Here's how the part is built. I have some questions about the finished solid (model axes, mm). Round coordinates to 2 decimals unless told otherwise and drop trailing zeros. Order: outer loops, then holes, each group sorted by start corner. A loop starts at its lowest first (then second) coordinate and runs counter-clockwise, first axis right, second up. Notation, with made-up numbers: (73, 40.5) - (103, 40.5) arc R30 ccw to (103, 74.5) - close; hole circle Ø1 at (-28, 14.25). An arc over 180 degrees is marked (long way). One line per item, written item: value.
from build123d import *

# Parameters (mm, degrees)
CYLINDER_R     = 5
CYLINDER_DEPTH = 500
BOX_W          = 45
BOX_H          = 45
BOX_DEPTH      = 350


with BuildPart() as screwhole:
    # Cylinder → Cylinder (new body)
    with BuildSketch(Plane(origin=(22.5, 22.5, -150), x_dir=(1, 0, 0), z_dir=(0, 0, 1))):
        Circle(CYLINDER_R)
    extrude(amount=CYLINDER_DEPTH)


with BuildPart() as screwedleg:
    # Box → Box (new body)
    with BuildSketch(Plane.XY):
        with Locations((22.5, 22.5)):
            Rectangle(BOX_W, BOX_H)
    extrude(amount=BOX_DEPTH)

    # Cut: cut ScrewHole
    add(screwhole.part, mode=Mode.SUBTRACT)


solid = screwedleg.part
Q1. If I drill on line 1 along Y through (x, z) = (22.5, 275.5); line 2 along X through (y, z) = (25, 75.5), over which ranges is the centre line in solid material (lowest first)?
Results list:
line 1: 0 to 17.5, 27.5 to 45
line 2: 0 to 18.17, 26.83 to 45
Q2. If we section it at C-C, the plane z = 140.5: Please give me the cut outline in (x, y).
Results list:
outline: (0, 0) - (45, 0) - (45, 45) - (0, 45) - close; hole circle Ø10 at (22.5, 22.5)
Q3. If we section it at A-A, the plane y = 22.5: Please give me the cut outline in (x, z).
Results list:
outline: (0, 0) - (17.5, 0) - (17.5, 350) - (0, 350) - close; (27.5, 0) - (45, 0) - (45, 350) - (27.5, 350) - close
